```python
from build123d import *

# Parameters (mm, degrees)
BOSS_EXTRUDE1_DEPTH = 8.89
SKETCH3_R           = 19.05
SKETCH3_R_2         = 3.175
CUT_EXTRUDE1_DEPTH  = 22.59
SKETCH4_R           = 19.05
BOSS_EXTRUDE3_DEPTH = 8.89


with BuildPart() as part:
    # Sketch1 → Boss-Extrude1 (new body)
    with BuildSketch(Plane(origin=(0, 0, 0), x_dir=(1, 0, 0), z_dir=(0, 1, 0))):
        with BuildLine():
            Line((40.8, 50.8), (-40.8, 50.8))
            ThreePointArc((-40.8, 50.8), (-47.871067812, 47.871067812), (-50.8, 40.8))
            Line((-50.8, 40.8), (-50.8, -40.8))
            ThreePointArc((-50.8, -40.8), (-47.871067812, -47.871067812), (-40.8, -50.8))
            Line((-40.8, -50.8), (40.8, -50.8))
            ThreePointArc((40.8, -50.8), (47.871067812, -47.871067812), (50.8, -40.8))
            Line((50.8, -40.8), (50.8, 40.8))
            ThreePointArc((50.8, 40.8), (47.871067812, 47.871067812), (40.8, 50.8))
        make_face()
    extrude(amount=BOSS_EXTRUDE1_DEPTH)

    # Sketch2 → Revolve1 (revolve)
    with BuildSketch(Plane.XY):
        Polygon((0, 8.89), (0, 21.59), (-25.4, 21.59), (-41.28, 8.89), align=None)
    revolve(axis=Axis((0, 8.89, 0), (0, 1, 0)))

    # Sketch3 → Cut-Extrude1 (cut, through all)
    with BuildSketch(Plane(origin=(0, 21.59, 0), x_dir=(1, 0, 0), z_dir=(0, 1, 0))):
        Circle(SKETCH3_R)
        with Locations((-38.1, 38.1)):
            Circle(SKETCH3_R_2)
        with Locations((38.1, 38.1)):
            Circle(SKETCH3_R_2)
        with Locations((38.1, -38.1)):
            Circle(SKETCH3_R_2)
        with Locations((-38.1, -38.1)):
            Circle(SKETCH3_R_2)
        with BuildLine():
            Line((-50.8, 19.05), (-50.8, -19.05))
            ThreePointArc((-50.8, -19.05), (-31.75, 0), (-50.8, 19.05))
        make_face()
        with BuildLine():
            Line((-19.05, 50.8), (19.05, 50.8))
            ThreePointArc((19.05, 50.8), (0, 31.75), (-19.05, 50.8))
        make_face()
        with BuildLine():
            Line((50.8, 19.05), (50.8, -19.05))
            ThreePointArc((50.8, -19.05), (31.75, 0), (50.8, 19.05))
        make_face()
        with BuildLine():
            Line((-19.05, -50.8), (19.05, -50.8))
            ThreePointArc((19.05, -50.8), (0, -31.75), (-19.05, -50.8))
        make_face()
    extrude(amount=-CUT_EXTRUDE1_DEPTH, mode=Mode.SUBTRACT)

    # Sketch4 → Boss-Extrude3 (add)
    with BuildSketch(Plane.XZ):
        Circle(SKETCH4_R)
    extrude(amount=-BOSS_EXTRUDE3_DEPTH)


solid = part.part
```
Work out the finished part from the listing and answer in its coordinate system (mm). A direction names the side the tool comes from. Give positions to 0.01 mm unless a question says otherwise; leave off trailing zeros. Loops run counter-clockwise (first coordinate to the right, second up) from the corner with the lowest first, then second, coordinate; pieces in that order, holes last. Notation, with made-up numbers: (-4.5, 78) - (17.5, 78) arc R22 ccw to (17.5, 86) - close; hole circle Ø9 at (-6, -6). An arc over 180 degrees is marked (long way). Use CSV: the item, a comma, the result in double quotes. Start each with the question number.
(1) Find the intervals of material crossed by L1, parallel to Z at x = 0, y = 14.25; L2, parallel to Z at x = -38.1, y = 4 (3 decimals), in increasing order.
(2) Find section C-C, the plane x = 0. Determine the outline of the cut face in (y, z), plus the area to 3 significant figures.
(3) Find section A-A, the plane y = 3. Determine the outline of the cut face in (x, z) (3 decimals), plus the area to 3 significant figures.
(4) Find section B-B, the plane z = 0. Determine the outline of the cut face in (x, y), plus the area to 3 significant figures.
(5) Determine the mould class of faces 4 (the face through (-50.8, 4, -30)), 5 (the face through (34.93, 4.51, -38.24)), 6 (the face through (-37, 8.89, 32)) for opening direction X: released by +X, released by -X, zero draft, split by the parting line, or undercut.
(6) Find section D-D, the plane y = 14.25. Determine the outline of the cut face in (x, z), plus the area to 3 significant figures.
(7) A tool of negligible diameter and unlimited length cuts with its end or side. For faces 1 (the face through (32, 8.89, -37)), 2 (the face through (-33, 8.89, -37)), 3 (the face through (36, 8.89, 32)), from which of +Z, -Z, +X, -X, +Y, -Y can it reach the whole face along a straight path? Write none if from no direction.
(8) Each of these flat-tipped pins is pushed along its axis until it touches: pin 1 (3 mm diameter, centred on x = -39, z = 21.5, fed in from +Y); pin 2 (2 mm diameter, centred on y = 7.5, z = 6, fed in from -X); pin 3 (8 mm diameter, centred on x = -10.5, y = 4, fed in from -Z). Where does it stop, or does it pass through?
Results found:
1,L1,"-31.75 to -19.05, 19.05 to 31.75"
1,L2,"-50.8 to -41.275, -34.925 to -14.199, 14.199 to 34.925, 41.275 to 50.8"
2,outline,"(0, -31.75) - (16.51, -31.75) - (21.59, -25.4) - (21.59, -19.05) - (8.89, -19.05) - (8.89, 19.05) - (21.59, 19.05) - (21.59, 25.4) - (16.51, 31.75) - (0, 31.75) - close"
2,area,"855 mm^2"
3,outline,"(-50.8, -40.8) arc R10 ccw to (-40.8, -50.8) - (-19.05, -50.8) arc R19.05 cw to (19.05, -50.8) - (40.8, -50.8) arc R10 ccw to (50.8, -40.8) - (50.8, -19.05) arc R19.05 cw to (50.8, 19.05) - (50.8, 40.8) arc R10 ccw to (40.8, 50.8) - (19.05, 50.8) arc R19.05 cw to (-19.05, 50.8) - (-40.8, 50.8) arc R10 ccw to (-50.8, 40.8) - (-50.8, 19.05) arc R19.05 cw to (-50.8, -19.05) - close; hole circle Ø6.35 at (-38.1, -38.1); hole circle Ø6.35 at (-38.1, 38.1); hole circle Ø6.35 at (38.1, -38.1); hole circle Ø6.35 at (38.1, 38.1)"
3,area,"7,830 mm^2"
4,outline,"(-31.75, 0) - (31.75, 0) - (31.75, 16.51) - (25.4, 21.59) - (19.05, 21.59) - (19.05, 8.89) - (-19.05, 8.89) - (-19.05, 21.59) - (-25.4, 21.59) - (-31.75, 16.51) - close"
4,area,"855 mm^2"
5,face 4,"released by -X"
5,face 5,"undercut"
5,face 6,"zero draft"
6,outline,"(-33.6, -8.18) arc R34.58 ccw to (-8.18, -33.6) arc R19.05 cw to (8.18, -33.6) arc R34.58 ccw to (33.6, -8.18) arc R19.05 cw to (33.6, 8.18) arc R34.58 ccw to (8.18, 33.6) arc R19.05 cw to (-8.18, 33.6) arc R34.58 ccw to (-33.6, 8.18) arc R19.05 cw to start; hole circle Ø38.1 at (0, 0)"
6,area,"2,490 mm^2"
7,face 1,"-Z, +X, +Y"
7,face 2,"-Z, -X, +Y"
7,face 3,"+Z, +X, +Y"
8,pin 1,"y = 8.89"
8,pin 2,"x = -33.08"
8,pin 3,"z = -38.44"
